Here's how the part is built. I have some questions about the finished solid (model axes, mm). A direction names the side the tool comes from. Round coordinates to 2 decimals unless told otherwise and drop trailing zeros. Order: outer loops, then holes, each group sorted by start corner. A loop starts at its lowest first (then second) coordinate and runs counter-clockwise, first axis right, second up.
```python
from build123d import *

# Parameters (mm, degrees)
SKETCH001_R       = 0.45
PAD001_DEPTH      = 6.25
PAD001_DEPTH_BACK = 3.5
SKETCH_R          = 5
PAD_DEPTH         = 12.5
FILLET_R          = 0.5


with BuildPart() as pad001:
    # Sketch001 → Pad001 (new body, two sides)
    with BuildSketch(Plane.XY.offset(0.5)) as pad001_sk:
        Circle(SKETCH001_R)
        with Locations((5, 0)):
            Circle(SKETCH001_R)
    extrude(amount=PAD001_DEPTH)
    extrude(pad001_sk.sketch, amount=-PAD001_DEPTH_BACK)


with BuildPart() as obj1:
    # Sketch → Pad (new body)
    with BuildSketch(Plane.XY.offset(0.1)):
        with Locations((2.5, 0)):
            Circle(SKETCH_R)
    extrude(amount=PAD_DEPTH)

    # Fillet
    fillet_edges = [obj1.edges().sort_by_distance(p)[0] for p in [
        (-2.5, 0, 0.1),
        (-2.5, 0, 12.6),
    ]]
    fillet(fillet_edges, radius=FILLET_R)

    # obj1: union Pad001
    add(pad001.part)


solid = obj1.part
```
1. I'm going to push flat-ended pins straight in: P1, Ø3, axis at x = -1, z = 2, coming from the +Y side; P2, Ø5, axis at x = 1.5, z = 6.5, coming from the -Y side; P3, Ø4, axis at y = 3, z = 7.5, coming from the -X side; P4, Ø1.5, axis at x = 1.5, z = 1.5, coming from the +Y side. Where does each tip first touch, or does it pass through?
Evaluation:
P1: stops at y = 4.58
P2: stops at y = -5
P3: stops at x = -2.4
P4: stops at y = 4.99
2. If we section it at B-B, the plane x = 2.5: Write out the boundary of the cut face in (y, z).
Evaluation:
outline: (-5, 0.6) arc R0.5 ccw to (-4.5, 0.1) - (4.5, 0.1) arc R0.5 ccw to (5, 0.6) - (5, 12.1) arc R0.5 ccw to (4.5, 12.6) - (-4.5, 12.6) arc R0.5 ccw to (-5, 12.1) - close
3. On a 3-axis mill with a long thin cutter (end or side, diameter ignored), from which of +Z, -Z, +X, -X, +Y, -Y can I reach the whole of each face in a straight line? I mean faces 1 (the flat face through (5, 0, -3)), 2 (the cylindrical face through (0.429, 0.135, -1.428)). Say none if no direction works.
Evaluation:
face 1: -Z, +X, -X, +Y, -Y
face 2: -Z
4. If we section it at D-D, the plane z = 7: Write out the boundary of the cut face in (x, y).
Evaluation:
outline: circle Ø10 at (2.5, 0)
5. If we mould it in two halves opening along X, with no side actions, what happens to faces 3 (the cylindrical face through (5.429, 0.135, -1.428)), 4 (the cylindrical face through (7.27, 1.5, 6.27)), 5 (the flat face through (2, 0, 12.6))? For each: released by +X, released by -X, zero draft, split by the parting line, or undercut.
Evaluation:
face 3: undercut
face 4: split by the parting line
face 5: zero draft
6. If we section it at A-A, the plane z = -1.5: Write out the boundary of the cut face in (x, y).
Evaluation:
outline: circle Ø0.9 at (0, 0); circle Ø0.9 at (5, 0)
7. If we section it at C-C, the plane y = 0: Write out the boundary of the cut face in (x, z).
Evaluation:
outline: (-2.5, 0.6) arc R0.5 ccw to (-2, 0.1) - (-0.45, 0.1) - (-0.45, -3) - (0.45, -3) - (0.45, 0.1) - (4.55, 0.1) - (4.55, -3) - (5.45, -3) - (5.45, 0.1) - (7, 0.1) arc R0.5 ccw to (7.5, 0.6) - (7.5, 12.1) arc R0.5 ccw to (7, 12.6) - (-2, 12.6) arc R0.5 ccw to (-2.5, 12.1) - close
8. I need wall thicknesses on probe 1 along Z at (x, y) = (2.5, 2.5); probe 2 along X at (y, z) = (-2, 1.25); probe 3 along Y at (x, z) = (5.5, 1.5). Which ranges of each line are inside material? Lowest first, please.
Evaluation:
probe 1: z = 0.1 to 12.6
probe 2: x = -2.08 to 7.08
probe 3: y = -4 to 4
